Geometry: final body of the model. Coordinates: model frame, mm. A direction names the side the tool comes from. Round coordinates to 2 decimals unless told otherwise and drop trailing zeros. Loops run counter-clockwise (first coordinate to the right, second up) from the corner with the lowest first, then second, coordinate; pieces in that order, holes last. Notation, with made-up numbers: (31, 45) - (71, 45) arc R19 ccw to (71, 68) - close; hole circle Ø10 at (61.5, 63). An arc over 180 degrees is marked (long way). Return JSON: item names as keys, results as strings. Group by question number.
1. Material intervals for probe 1 along X at (y, z) = (43, 6.25); probe 2 along Y at (x, z) = (24, 21); probe 3 along X at (y, z) = (26.5, 1.4), sorted ascending.
2. Section C-C on z = 6.25. Count the separate pieces of the cut face and the enclosed holes in it, and give its area (3 significant figures).
3. Set-up query: faces 5 (the face through (-22.37, 28.9, 6.34)), 6 (the face through (23, -14, 22)), 7 (the face through (-17.796, 45.975, 6.233)). Return all of +Z, -Z, +X, -X, +Y, -Y with unobstructed straight access to the full face (end or side cutting, diameter ignored); none if empty.
4. Draft query along X for faces 1 (the face through (15.889, 49.066, 20.384)), 2 (the face through (-0.2, 52.38, 15.98)), 3 (the face through (27.074, 17.71, 24.034)), 4 (the face through (-12, 41, 14)). Return one class per face: +X half, -X half, draft (parallel to the pull), parting line (faces both ways), or undercut.
5. First-contact query: pin 1 Ø2 at (x, y) = (-13.5, 37) entering from -Z; pin 2 Ø1 at (x, y) = (27.5, -19) entering from -Z; pin 3 Ø3.5 at (x, z) = (26, 18) entering from -Y. Flat tips, straight axial feed; report the tip coordinate or a pass-through.
6. Section B-B on y = -5.5. Return loops of the section in (x, z), and give its area (3 significant figures).
from build123d import *

# Parameters (mm, degrees)
BOSS_EXTRUDE1_DEPTH = 32
CUT_EXTRUDE1_START  = 52.5
SKETCH2_W           = 30
SKETCH2_H           = 8.5
CUT_EXTRUDE1_DEPTH  = 25
CUT_EXTRUDE3_START  = 20
SKETCH3_W           = 30
SKETCH3_H           = 14
CUT_EXTRUDE3_DEPTH  = 25
CUT_EXTRUDE4_START  = 32
SKETCH4_W           = 10
SKETCH4_H           = 5
CUT_EXTRUDE4_DEPTH  = 21.5
CUT_EXTRUDE5_START  = 30
SKETCH5_W           = 8
SKETCH5_H           = 20
SKETCH5_W_2         = 13
SKETCH5_H_2         = 38
CUT_EXTRUDE5_DEPTH  = 60
SKETCH6_W           = 14
SKETCH6_H           = 27
CUT_EXTRUDE6_DEPTH  = 25
CUT_EXTRUDE7_START  = -30
SKETCH7_W           = 16
SKETCH7_H           = 40
CUT_EXTRUDE7_DEPTH  = 5
CUT_EXTRUDE8_START  = 30
SKETCH7_2_W         = 16
SKETCH7_2_H         = 40
CUT_EXTRUDE8_DEPTH  = 5
CUT_EXTRUDE9_START  = -10
SKETCH8_W           = 8
SKETCH8_H           = 20
CUT_EXTRUDE9_DEPTH  = 15
CUT_EXTRUDE10_START = -10
SKETCH9_W           = 8
SKETCH9_H           = 20
CUT_EXTRUDE10_DEPTH = 15
CUT_EXTRUDE11_START = -14
SKETCH11_W          = 16.7
SKETCH11_H          = 27
CUT_EXTRUDE11_DEPTH = 15
CUT_EXTRUDE12_START = -14
SKETCH12_W          = 16.7
SKETCH12_H          = 27
CUT_EXTRUDE12_DEPTH = 16
CUT_EXTRUDE13_DEPTH = 31
CUT_EXTRUDE14_DEPTH = 31
BOSS_EXTRUDE2_START = 45
SKETCH16_R          = 3.5
SKETCH16_R_2        = 1.25
BOSS_EXTRUDE2_DEPTH = 5.5
CUT_EXTRUDE15_START = -10
SKETCH17_R          = 1.1
CUT_EXTRUDE15_DEPTH = 10
FILLET3_R           = 3
CHAMFER1_SIZE       = 2
SKETCH18_R          = 1.6
CUT_EXTRUDE16_DEPTH = 6
CUT_EXTRUDE17_START = 13
SKETCH19_W          = 3
SKETCH19_H          = 7.5
CUT_EXTRUDE17_DEPTH = 19
BOSS_EXTRUDE4_START = -17.5
SKETCH21_W          = 2
SKETCH21_H          = 5
BOSS_EXTRUDE4_DEPTH = 3
BOSS_EXTRUDE5_START = 13
SKETCH22_W          = 3
SKETCH22_H          = 5
BOSS_EXTRUDE5_DEPTH = 3
CUT_EXTRUDE18_START = 15.3
CUT_EXTRUDE18_DEPTH = 6
CUT_EXTRUDE20_DEPTH = 42
CUT_EXTRUDE21_START = 49.5
CUT_EXTRUDE21_DEPTH = 10
BOSS_EXTRUDE6_START = 52.5
SKETCH26_R          = 1.25
BOSS_EXTRUDE6_DEPTH = 10


with BuildPart() as part:
    # Sketch1 → Boss-Extrude1 (new body)
    with BuildSketch(Plane.XY):
        Polygon((-30, 17.5), (-15, 52.5), (15, 52.5), (30, 17.5), (30, -17.5), (20, -17.5), (20, 15.44742298), (8.40603842, 42.5), (-8.40603842, 42.5), (-20, 15.44742298), (-20, -17.5), (-30, -17.5), align=None)
    extrude(amount=BOSS_EXTRUDE1_DEPTH)

    # Sketch2 → Cut-Extrude1 (cut)
    with BuildSketch(Plane(origin=(0, 0, 0), x_dir=(1, 0, 0), z_dir=(0, 1, 0)).offset(CUT_EXTRUDE1_START)):
        with Locations((0, -6.25)):
            Rectangle(SKETCH2_W, SKETCH2_H)
    extrude(amount=-CUT_EXTRUDE1_DEPTH, mode=Mode.SUBTRACT)

    # Sketch3 → Cut-Extrude3 (cut)
    with BuildSketch(Plane(origin=(0, 0, 0), x_dir=(1, 0, 0), z_dir=(0, 1, 0)).offset(CUT_EXTRUDE3_START)):
        with Locations((0, -7)):
            Rectangle(SKETCH3_W, SKETCH3_H)
        with BuildLine():
            Line((18.37, -10.25), (-18.37, -10.25))
            ThreePointArc((-18.37, -10.25), (-22.37, -6.25), (-18.37, -2.25))
            Line((-18.37, -2.25), (18.37, -2.25))
            ThreePointArc((18.37, -2.25), (22.37, -6.25), (18.37, -10.25))
        make_face()
    extrude(amount=CUT_EXTRUDE3_DEPTH, mode=Mode.SUBTRACT)

    # Sketch4 → Cut-Extrude4 (cut)
    with BuildSketch(Plane.XY.offset(CUT_EXTRUDE4_START)):
        with Locations((0, 45)):
            Rectangle(SKETCH4_W, SKETCH4_H)
    extrude(amount=-CUT_EXTRUDE4_DEPTH, mode=Mode.SUBTRACT)

    # Sketch5 → Cut-Extrude5 (cut)
    with BuildSketch(Plane(origin=(0, 0, 0), x_dir=(0, 0, -1), z_dir=(1, 0, 0)).offset(CUT_EXTRUDE5_START)):
        with Locations((-23.5, 3.5)):
            Rectangle(SKETCH5_W, SKETCH5_H)
        with Locations((-6.5, 1.5)):
            Rectangle(SKETCH5_W_2, SKETCH5_H_2)
    extrude(amount=-CUT_EXTRUDE5_DEPTH, mode=Mode.SUBTRACT)

    # Sketch6 → Cut-Extrude6 (cut, symmetric)
    with BuildSketch(Plane(origin=(0, 0, 0), x_dir=(0, 0, -1), z_dir=(1, 0, 0))):
        with Locations((-25, 3.5)):
            Rectangle(SKETCH6_W, SKETCH6_H)
    extrude(amount=CUT_EXTRUDE6_DEPTH, both=True, mode=Mode.SUBTRACT)

    # Sketch7 → Cut-Extrude7 (cut)
    with BuildSketch(Plane(origin=(0, 0, 0), x_dir=(0, 0, -1), z_dir=(1, 0, 0)).offset(CUT_EXTRUDE7_START)):
        with Locations((-8, 2.5)):
            Rectangle(SKETCH7_W, SKETCH7_H)
    extrude(amount=CUT_EXTRUDE7_DEPTH, mode=Mode.SUBTRACT)

    # Sketch7<2> → Cut-Extrude8 (cut)
    with BuildSketch(Plane(origin=(0, 0, 0), x_dir=(0, 0, -1), z_dir=(1, 0, 0)).offset(CUT_EXTRUDE8_START)):
        with Locations((-8, 2.5)):
            Rectangle(SKETCH7_2_W, SKETCH7_2_H)
    extrude(amount=-CUT_EXTRUDE8_DEPTH, mode=Mode.SUBTRACT)

    # Sketch8 → Cut-Extrude9 (cut)
    with BuildSketch(Plane(origin=(-40.872484783, 17.516779193, 0), x_dir=(0, 0, 1), z_dir=(-0.9191450300180579, 0.3939192985791677, 0)).offset(CUT_EXTRUDE9_START)):
        with Locations((20.8, 23.306891833)):
            Rectangle(SKETCH8_W, SKETCH8_H)
    extrude(amount=-CUT_EXTRUDE9_DEPTH, mode=Mode.SUBTRACT)

    # Sketch9 → Cut-Extrude10 (cut)
    with BuildSketch(Plane(origin=(40.872484783, 17.516779193, 0), x_dir=(0, 0, -1), z_dir=(0.9191450300180579, 0.3939192985791677, 0)).offset(CUT_EXTRUDE10_START)):
        with Locations((-20.8, 23.306891833)):
            Rectangle(SKETCH9_W, SKETCH9_H)
    extrude(amount=-CUT_EXTRUDE10_DEPTH, mode=Mode.SUBTRACT)

    # Sketch11 → Cut-Extrude11 (cut)
    with BuildSketch(Plane(origin=(-40.872484783, 17.516779193, 0), x_dir=(0, 0, 1), z_dir=(-0.9191450300180579, 0.3939192985791677, 0)).offset(CUT_EXTRUDE11_START)):
        with Locations((23.65, 23.306891833)):
            Rectangle(SKETCH11_W, SKETCH11_H)
    extrude(amount=-CUT_EXTRUDE11_DEPTH, mode=Mode.SUBTRACT)

    # Sketch12 → Cut-Extrude12 (cut)
    with BuildSketch(Plane(origin=(40.872484783, 17.516779193, 0), x_dir=(0, 0, -1), z_dir=(0.9191450300180579, 0.3939192985791677, 0)).offset(CUT_EXTRUDE12_START)):
        with Locations((-23.65, 23.306891833)):
            Rectangle(SKETCH12_W, SKETCH12_H)
    extrude(amount=-CUT_EXTRUDE12_DEPTH, mode=Mode.SUBTRACT)

    # Sketch13 → Cut-Extrude13 (cut, symmetric)
    with BuildSketch(Plane(origin=(0, 0, 0), x_dir=(0, 0, -1), z_dir=(1, 0, 0))):
        Polygon((-32, 52.5), (-26, 52.5), (-32, -17.5), align=None)
    extrude(amount=CUT_EXTRUDE13_DEPTH, both=True, mode=Mode.SUBTRACT)

    # Sketch14 → Cut-Extrude14 (cut, symmetric)
    with BuildSketch(Plane(origin=(0, 0, 0), x_dir=(0, 0, -1), z_dir=(1, 0, 0))):
        Polygon((-16, 52.5), (-26, 52.5), (-26.571475939, 45.832780711), align=None)
    extrude(amount=CUT_EXTRUDE14_DEPTH, both=True, mode=Mode.SUBTRACT)

    # Sketch16 → Boss-Extrude2 (add)
    # profile 1 of 2: a face of its own
    with BuildSketch(Plane(origin=(0, 0, 0), x_dir=(1, 0, 0), z_dir=(0, 1, 0)).offset(BOSS_EXTRUDE2_START)):
        with Locations(Location((18.37, -6.25, 0), (0, 0, 270))):
            Circle(SKETCH16_R)
        with Locations(Location((18.37, -6.25, 0), (0, 0, 270))):
            Circle(SKETCH16_R_2, mode=Mode.SUBTRACT)
    # profile 2 of 2: a face of its own
    with BuildSketch(Plane(origin=(0, 0, 0), x_dir=(1, 0, 0), z_dir=(0, 1, 0)).offset(BOSS_EXTRUDE2_START)):
        with Locations(Location((-18.37, -6.25, 0), (0, 0, 270))):
            Circle(SKETCH16_R)
        with Locations(Location((-18.37, -6.25, 0), (0, 0, 270))):
            Circle(SKETCH16_R_2, mode=Mode.SUBTRACT)
    extrude(amount=-BOSS_EXTRUDE2_DEPTH)

    # Sketch17 → Cut-Extrude15 (cut)
    with BuildSketch(Plane(origin=(0, 3.449230214, 40.241019165), x_dir=(1, 0, 0), z_dir=(0, 0.08540114134643577, 0.9963466490417511)).offset(CUT_EXTRUDE15_START)):
        with Locations(Location((-27, -16.168902881, 0), (0, 0, 90))):
            Circle(SKETCH17_R)
        with Locations(Location((-26, 15.831097119, 0), (0, 0, 90))):
            Circle(SKETCH17_R)
        with Locations(Location((27, -16.168902881, 0), (0, 0, 90))):
            Circle(SKETCH17_R)
        with Locations(Location((26, 15.831097119, 0), (0, 0, 90))):
            Circle(SKETCH17_R)
    extrude(amount=-CUT_EXTRUDE15_DEPTH, mode=Mode.SUBTRACT)

    # Fillet3
    fillet3_edges = [part.edges().sort_by_distance(p)[0] for p in [
        (30, 17.5, 22.5),
        (-30, 17.5, 22.5),
        (0, 52.5, 16),
        (16.428689848, 49.166390355, 21.28573797),
        (-16.428689848, 49.166390355, 21.28573797),
    ]]
    fillet(fillet3_edges, radius=FILLET3_R)

    # Chamfer1
    chamfer1_edges = [part.edges().sort_by_distance(p)[0] for p in [
        (0, 52.5, 0),
    ]]
    chamfer(chamfer1_edges, length=CHAMFER1_SIZE - 0.0001)  # a hair under: the kernel refuses the full size

    # Sketch18 → Cut-Extrude16 (cut)
    with BuildSketch(Plane.XY):
        with Locations(Location((18, 26.5, 0), (0, 0, 283.370675639))):
            Circle(SKETCH18_R)
        with Locations(Location((-18, 26.5, 0), (0, 0, 180))):
            Circle(SKETCH18_R)
    extrude(amount=CUT_EXTRUDE16_DEPTH, mode=Mode.SUBTRACT)

    # Sketch19 → Cut-Extrude17 (cut)
    with BuildSketch(Plane.XY.offset(CUT_EXTRUDE17_START)):
        with Locations((-21.5, -13.75)):
            Rectangle(SKETCH19_W, SKETCH19_H)
        with Locations((21.5, -13.75)):
            Rectangle(SKETCH19_W, SKETCH19_H)
    extrude(amount=CUT_EXTRUDE17_DEPTH, mode=Mode.SUBTRACT)

    # Sketch21 → Boss-Extrude4 (add)
    with BuildSketch(Plane(origin=(0, 0, 0), x_dir=(1, 0, 0), z_dir=(0, 1, 0)).offset(BOSS_EXTRUDE4_START)):
        with Locations((-27, -23.5)):
            Rectangle(SKETCH21_W, SKETCH21_H)
        with Locations((27, -23.5)):
            Rectangle(SKETCH21_W, SKETCH21_H)
    extrude(amount=-BOSS_EXTRUDE4_DEPTH)

    # Sketch22 → Boss-Extrude5 (add)
    with BuildSketch(Plane.XY.offset(BOSS_EXTRUDE5_START)):
        with Locations((-21.5, 13)):
            Rectangle(SKETCH22_W, SKETCH22_H)
        with Locations((21.5, 13)):
            Rectangle(SKETCH22_W, SKETCH22_H)
    extrude(amount=-BOSS_EXTRUDE5_DEPTH)

    # Sketch23 → Cut-Extrude18 (cut)
    with BuildSketch(Plane.XY.offset(CUT_EXTRUDE18_START)):
        Polygon((-16.063333209, 17.5538661), (-19.545605261, 19.046268408), (-8.909784199, 43.863184218), (-5.427512148, 42.37078191), align=None)
        Polygon((16.063333209, 17.5538661), (19.545605261, 19.046268408), (8.909784199, 43.863184218), (5.427512148, 42.37078191), align=None)
    extrude(amount=-CUT_EXTRUDE18_DEPTH, mode=Mode.SUBTRACT)

    # Sketch24 → Cut-Extrude20 (cut)
    with BuildSketch(Plane.XY):
        Polygon((-20, 15.44742298), (-20, 17.986014016), (-19.076948331, 20.139801243), (-18.160478874, 19.739638942), align=None)
        Polygon((20, 15.44742298), (18.160478874, 19.739638942), (19.076948331, 20.139801243), (20, 17.986014016), align=None)
    extrude(amount=CUT_EXTRUDE20_DEPTH, mode=Mode.SUBTRACT)

    # Sketch25 → Cut-Extrude21 (cut)
    with BuildSketch(Plane(origin=(0, 0, 0), x_dir=(1, 0, 0), z_dir=(0, 1, 0)).offset(CUT_EXTRUDE21_START)):
        with BuildLine():
            Line((-15, -7.195039682), (-15, -5.304960318))
            ThreePointArc((-15, -5.304960318), (-14.87, -6.25), (-15, -7.195039682))
        make_face()
        with BuildLine():
            Line((15, -7.195039682), (15, -5.304960318))
            ThreePointArc((15, -5.304960318), (14.87, -6.25), (15, -7.195039682))
        make_face()
    extrude(amount=-CUT_EXTRUDE21_DEPTH, mode=Mode.SUBTRACT)

    # Sketch26 → Boss-Extrude6 (add)
    # profile 1 of 2: a face of its own
    with BuildSketch(Plane(origin=(0, 0, 0), x_dir=(1, 0, 0), z_dir=(0, 1, 0)).offset(BOSS_EXTRUDE6_START)):
        with BuildLine():
            Line((-14.74078782, -9.68930501), (-14.74078782, -2.81069499))
            ThreePointArc((-14.74078782, -2.81069499), (-23.37, -6.25), (-14.74078782, -9.68930501))
        make_face()
        with Locations(Location((-18.37, -6.25, 0), (0, 0, 270))):
            Circle(SKETCH26_R, mode=Mode.SUBTRACT)
    # profile 2 of 2: a face of its own
    with BuildSketch(Plane(origin=(0, 0, 0), x_dir=(1, 0, 0), z_dir=(0, 1, 0)).offset(BOSS_EXTRUDE6_START)):
        with BuildLine():
            Line((15.237989525, -10.147500531), (15.237989525, -2.352499469))
            ThreePointArc((15.237989525, -2.352499469), (23.37, -6.25), (15.237989525, -10.147500531))
        make_face()
        with Locations(Location((18.37, -6.25, 0), (0, 0, 270))):
            Circle(SKETCH26_R, mode=Mode.SUBTRACT)
    extrude(amount=-BOSS_EXTRUDE6_DEPTH)


solid = part.part
Taken from the geometry:
{
 "1": {"probe 1": "-23.37 to -19.62, -17.12 to -14.74, 15 to 17.12, 19.62 to 23.37", "probe 2": "-17.5 to -10, 17 to 20.96, 21.35 to 24.76", "probe 3": "-26.14 to -19.6, -16.4 to -15.26, 15.26 to 16.4, 19.6 to 26.14"},
 "2": {"separate pieces": "6", "enclosed holes": "0", "area": "230 mm2"},
 "3": {"face 5": "-Y", "face 6": "+Z, -Z, -Y", "face 7": "+Y"},
 "4": {"face 1": "+X half", "face 2": "draft", "face 3": "undercut", "face 4": "undercut"},
 "5": {"pin 1": "z = 14", "pin 2": "z = 21", "pin 3": "y = -17.5"},
 "6": {"outline": "(-30, 16) - (-25, 16) - (-25, 13) - (-20, 13) - (-20, 18) - (-25, 18) - (-25, 19.5) - (-30, 19.5) - close; (-30, 27.5) - (-25, 27.5) - (-25, 30.97) - (-30, 30.97) - close; (20, 13) - (25, 13) - (25, 16) - (30, 16) - (30, 19.5) - (25, 19.5) - (25, 18) - (20, 18) - close; (25, 27.5) - (30, 27.5) - (30, 30.97) - (25, 30.97) - close", "area": "120 mm2"}
}
